Here's how the part is built. I have some questions about the finished solid (model axes, mm). Face numbers are marked on the shaded views. A direction names the side the tool comes from. Coordinates: 2 decimals unless noted, no trailing zeros. Write each loop counter-clockwise with the first axis right and the second up, starting at its lowest first coordinate (ties: lowest second). Pieces come first, ordered by that corner, then holes. Notation, with made-up numbers: (3, 60.5) -> (32, 60.5) arc R26 ccw to (32, 83.5) -> close; hole circle Ø8 at (47, -19). An arc over 180 degrees is marked (long way). Use CSV: the item, a comma, the result in double quotes. Start each with the question number.
```python
from build123d import *
from build123d.topology import SkipClean

# Parameters (mm, degrees)
BOSS_EXTRUDE1_DEPTH      = 17
BOSS_EXTRUDE1_DEPTH_BACK = 6
SKETCH1_R                = 11
SKETCH1_R_2              = 3.2
CUT_EXTRUDE1_START       = -10
CUT_EXTRUDE1_DEPTH       = 10


with BuildPart() as part:
    # Sketch1 → Boss-Extrude1 (new, two sides: drawn at the far end of the back side and taken through both)
    # profile 1 of 9: a face of its own
    with BuildSketch(Plane(origin=(0, 0, 0), x_dir=(1, 0, 0), z_dir=(0, 1, 0)).offset(-BOSS_EXTRUDE1_DEPTH_BACK)):
        Circle(SKETCH1_R)
        with Locations(Location((0, 0, 0), (0, 0, 270))):
            Circle(SKETCH1_R_2, mode=Mode.SUBTRACT)
    # profile 2 of 9: a face of its own
    with BuildSketch(Plane(origin=(0, 0, 0), x_dir=(1, 0, 0), z_dir=(0, 1, 0)).offset(-BOSS_EXTRUDE1_DEPTH_BACK)):
        with BuildLine():
            ThreePointArc((-10.583005244, 3), (-14.702730308, 2.689388484), (-18.472953202, 1))
            ThreePointArc((-18.472953202, 1), (-18.5, 0), (-18.472953202, -1))
            ThreePointArc((-18.472953202, -1), (-14.702730308, -2.689388484), (-10.583005244, -3))
            ThreePointArc((-10.583005244, -3), (-11, 0), (-10.583005244, 3))
        make_face()
    # profile 3 of 9: a face of its own
    with BuildSketch(Plane(origin=(0, 0, 0), x_dir=(1, 0, 0), z_dir=(0, 1, 0)).offset(-BOSS_EXTRUDE1_DEPTH_BACK)):
        with BuildLine():
            ThreePointArc((-5.36199443, 9.604635117), (-8.494715469, 12.298085137), (-12.355243696, 13.769457259))
            ThreePointArc((-12.355243696, 13.769457259), (-13.081475452, 13.081475452), (-13.769457259, 12.355243696))
            ThreePointArc((-13.769457259, 12.355243696), (-12.298085137, 8.494715469), (-9.604635117, 5.36199443))
            ThreePointArc((-9.604635117, 5.36199443), (-7.778174593, 7.778174593), (-5.36199443, 9.604635117))
        make_face()
    # profile 4 of 9: a face of its own
    with BuildSketch(Plane(origin=(0, 0, 0), x_dir=(1, 0, 0), z_dir=(0, 1, 0)).offset(-BOSS_EXTRUDE1_DEPTH_BACK)):
        with BuildLine():
            ThreePointArc((3, 10.583005244), (2.689388484, 14.702730308), (1, 18.472953202))
            ThreePointArc((1, 18.472953202), (0, 18.5), (-1, 18.472953202))
            ThreePointArc((-1, 18.472953202), (-2.689388484, 14.702730308), (-3, 10.583005244))
            ThreePointArc((-3, 10.583005244), (0, 11), (3, 10.583005244))
        make_face()
    # profile 5 of 9: a face of its own
    with BuildSketch(Plane(origin=(0, 0, 0), x_dir=(1, 0, 0), z_dir=(0, 1, 0)).offset(-BOSS_EXTRUDE1_DEPTH_BACK)):
        with BuildLine():
            ThreePointArc((9.604635117, 5.36199443), (12.298085137, 8.494715469), (13.769457259, 12.355243696))
            ThreePointArc((13.769457259, 12.355243696), (13.081475452, 13.081475452), (12.355243696, 13.769457259))
            ThreePointArc((12.355243696, 13.769457259), (8.494715469, 12.298085137), (5.36199443, 9.604635117))
            ThreePointArc((5.36199443, 9.604635117), (7.778174593, 7.778174593), (9.604635117, 5.36199443))
        make_face()
    # profile 6 of 9: a face of its own
    with BuildSketch(Plane(origin=(0, 0, 0), x_dir=(1, 0, 0), z_dir=(0, 1, 0)).offset(-BOSS_EXTRUDE1_DEPTH_BACK)):
        with BuildLine():
            ThreePointArc((18.472953202, -1), (18.493237064, -0.500182849), (18.5, 0))
            ThreePointArc((18.5, 0), (18.493237064, 0.500182849), (18.472953202, 1))
            ThreePointArc((18.472953202, 1), (14.702730308, 2.689388484), (10.583005244, 3))
            ThreePointArc((10.583005244, 3), (10.895252583, 1.514421063), (11, 0))
            ThreePointArc((11, 0), (10.895252583, -1.514421063), (10.583005244, -3))
            ThreePointArc((10.583005244, -3), (14.702730308, -2.689388484), (18.472953202, -1))
        make_face()
    # profile 7 of 9: a face of its own
    with BuildSketch(Plane(origin=(0, 0, 0), x_dir=(1, 0, 0), z_dir=(0, 1, 0)).offset(-BOSS_EXTRUDE1_DEPTH_BACK)):
        with BuildLine():
            ThreePointArc((12.355243696, -13.769457259), (13.081475452, -13.081475452), (13.769457259, -12.355243696))
            ThreePointArc((13.769457259, -12.355243696), (12.298085137, -8.494715469), (9.604635117, -5.36199443))
            ThreePointArc((9.604635117, -5.36199443), (7.778174593, -7.778174593), (5.36199443, -9.604635117))
            ThreePointArc((5.36199443, -9.604635117), (8.494715469, -12.298085137), (12.355243696, -13.769457259))
        make_face()
    # profile 8 of 9: a face of its own
    with BuildSketch(Plane(origin=(0, 0, 0), x_dir=(1, 0, 0), z_dir=(0, 1, 0)).offset(-BOSS_EXTRUDE1_DEPTH_BACK)):
        with BuildLine():
            ThreePointArc((-1, -18.472953202), (0, -18.5), (1, -18.472953202))
            ThreePointArc((1, -18.472953202), (2.689388484, -14.702730308), (3, -10.583005244))
            ThreePointArc((3, -10.583005244), (0, -11), (-3, -10.583005244))
            ThreePointArc((-3, -10.583005244), (-2.689388484, -14.702730308), (-1, -18.472953202))
        make_face()
    # profile 9 of 9: a face of its own
    with BuildSketch(Plane(origin=(0, 0, 0), x_dir=(1, 0, 0), z_dir=(0, 1, 0)).offset(-BOSS_EXTRUDE1_DEPTH_BACK)):
        with BuildLine():
            ThreePointArc((-13.769457259, -12.355243696), (-13.081475452, -13.081475452), (-12.355243696, -13.769457259))
            ThreePointArc((-12.355243696, -13.769457259), (-8.494715469, -12.298085137), (-5.36199443, -9.604635117))
            ThreePointArc((-5.36199443, -9.604635117), (-7.778174593, -7.778174593), (-9.604635117, -5.36199443))
            ThreePointArc((-9.604635117, -5.36199443), (-12.298085137, -8.494715469), (-13.769457259, -12.355243696))
        make_face()
    extrude(amount=BOSS_EXTRUDE1_DEPTH + BOSS_EXTRUDE1_DEPTH_BACK)

    # Sketch1_7 → Cut-Extrude1 (cut)
    with SkipClean():  # the faces are left unmerged after this step: merging them gives an invalid solid
        with BuildSketch(Plane(origin=(0, 0, 0), x_dir=(1, 0, 0), z_dir=(0, 1, 0)).offset(CUT_EXTRUDE1_START)):
            with BuildLine():
                ThreePointArc((18.472953202, -1), (18.493237064, -0.500182849), (18.5, 0))
                ThreePointArc((18.5, 0), (18.493237064, 0.500182849), (18.472953202, 1))
                ThreePointArc((18.472953202, 1), (14.702730308, 2.689388484), (10.583005244, 3))
                ThreePointArc((10.583005244, 3), (10.895252583, 1.514421063), (11, 0))
                ThreePointArc((11, 0), (10.895252583, -1.514421063), (10.583005244, -3))
                ThreePointArc((10.583005244, -3), (14.702730308, -2.689388484), (18.472953202, -1))
            make_face()
            with BuildLine():
                ThreePointArc((3, 10.583005244), (2.689388484, 14.702730308), (1, 18.472953202))
                ThreePointArc((1, 18.472953202), (0, 18.5), (-1, 18.472953202))
                ThreePointArc((-1, 18.472953202), (-2.689388484, 14.702730308), (-3, 10.583005244))
                ThreePointArc((-3, 10.583005244), (0, 11), (3, 10.583005244))
            make_face()
            with BuildLine():
                ThreePointArc((-10.583005244, 3), (-14.702730308, 2.689388484), (-18.472953202, 1))
                ThreePointArc((-18.472953202, 1), (-18.5, 0), (-18.472953202, -1))
                ThreePointArc((-18.472953202, -1), (-14.702730308, -2.689388484), (-10.583005244, -3))
                ThreePointArc((-10.583005244, -3), (-11, 0), (-10.583005244, 3))
            make_face()
            with BuildLine():
                ThreePointArc((-1, -18.472953202), (0, -18.5), (1, -18.472953202))
                ThreePointArc((1, -18.472953202), (2.689388484, -14.702730308), (3, -10.583005244))
                ThreePointArc((3, -10.583005244), (0, -11), (-3, -10.583005244))
                ThreePointArc((-3, -10.583005244), (-2.689388484, -14.702730308), (-1, -18.472953202))
            make_face()
        extrude(amount=CUT_EXTRUDE1_DEPTH, mode=Mode.SUBTRACT)


solid = part.part
```
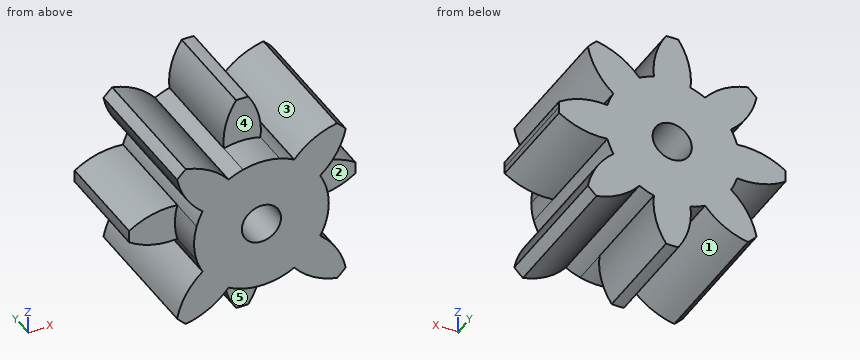
Item 1: I want a section at D-D on y = -3.5. Please give me the cut outline in (x, z), then the cut area to 3 significant figures.
Item 2: If I drill on line 1 along X through (y, z) = (10.5, 11); line 2 along Y through (x, z) = (-2, 14); line 3 along X through (y, z) = (12.5, -12), over which ranges is the centre line in solid material (lowest first)?
Item 3: I want a section at C-C on x = 13. Please give me the cut outline in (y, z).
Item 4: I want a section at B-B on x = 0. Please give me the cut outline in (y, z), then the cut area to 3 significant figures.
Item 5: I'm going to push flat-ended pins straight in: pin 1 (5 mm diameter, centred on y = 10, z = 9.5, fed in from -X); pin 2 (1.8 mm diameter, centred on x = 15.5, z = -1, fed in from -Y); pin 3 (1 mm diameter, centred on x = -8, y = 5, fed in from +Z). Where does each tip first touch, or does it pass through?
Item 6: Which directions (+Z, -Z, +X, -X, +Y, -Y) give clear straight access to the entire face, cutting with the end or side of a thin tool? Please do the marked faces 1, 2, 3, 4 and 5.
Geometry says:
1,outline,"(-13.77, -12.36) arc R18.5 ccw to (-12.36, -13.77) arc R12 ccw to (-5.36, -9.6) arc R11 ccw to (5.36, -9.6) arc R12 ccw to (12.36, -13.77) arc R18.5 ccw to (13.77, -12.36) arc R12 ccw to (9.6, -5.36) arc R11 ccw to (9.6, 5.36) arc R12 ccw to (13.77, 12.36) arc R18.5 ccw to (12.36, 13.77) arc R12 ccw to (5.36, 9.6) arc R11 ccw to (-5.36, 9.6) arc R12 ccw to (-12.36, 13.77) arc R18.5 ccw to (-13.77, 12.36) arc R12 ccw to (-9.6, 5.36) arc R11 ccw to (-9.6, -5.36) arc R12 ccw to start; hole circle Ø6.4 at (0, 0)"
1,area,"499 mm2"
2,line 1,"-13.42 to -6.71, -3.03 to 3.03, 6.71 to 13.42"
2,line 2,"0 to 17"
2,line 3,"-13.7 to -8.02, -3.05 to 3.05, 8.02 to 13.7"
3,outline,"(-6, -13.16) -> (17, -13.16) -> (17, -9.87) -> (-6, -9.87) -> close; (-6, 9.87) -> (17, 9.87) -> (17, 13.16) -> (-6, 13.16) -> close; (0, -2.99) -> (17, -2.99) -> (17, 2.99) -> (0, 2.99) -> close"
4,outline,"(-6, -11) -> (0, -11) -> (0, -18.5) -> (17, -18.5) -> (17, -3.2) -> (-6, -3.2) -> close; (-6, 3.2) -> (17, 3.2) -> (17, 18.5) -> (0, 18.5) -> (0, 11) -> (-6, 11) -> close"
4,area,"614 mm2"
5,pin 1,"x = -13.7"
5,pin 2,"y = 0"
5,pin 3,"z = 12.3"
6,face 1,"-Z, +Y, -Y"
6,face 2,"+X, -Y"
6,face 3,"+Z, +Y, -Y"
6,face 4,"+Z, -Y"
6,face 5,"-Z, -Y"
